CAD build for the part. Positions are in the model's coordinates, mm. A direction names the side the tool comes from. Round coordinates to 2 decimals unless told otherwise and drop trailing zeros. Loops run counter-clockwise (first coordinate to the right, second up) from the corner with the lowest first, then second, coordinate; pieces in that order, holes last. Notation, with made-up numbers: M 17.5,31 L 35.5,31 A15 cw 35.5,46 Z; hole C 88.5,-32 d5. An arc over 180 degrees is marked long. Put each result on its own line as item: value. Start each with the question number.
from build123d import *

# Parameters (mm, degrees)
BOSS_EXTRUDE1_DEPTH      = 15.5
BOSS_EXTRUDE1_DEPTH_BACK = 15.5
SKETCH1_W                = 63.5
SKETCH1_H                = 58.5
SHELL1_T                 = 3
SKETCH2_W                = 16
SKETCH2_H                = 52
CUT_EXTRUDE1_DEPTH       = 39.5
SKETCH3_W                = 53.5
SKETCH3_H                = 31
CUT_EXTRUDE2_DEPTH       = 39.5
BOSS_EXTRUDE2_START      = -15.5
SKETCH4_R                = 1.6
BOSS_EXTRUDE2_DEPTH      = 3
FILLET1_R                = 3.5
FILLET2_R                = 1


with BuildPart() as part:
    # Sketch1 → Boss-Extrude1 (new, two sides: drawn at the far end of the back side and taken through both)
    with BuildSketch(Plane(origin=(0, 0, 0), x_dir=(1, 0, 0), z_dir=(0, 1, 0)).offset(-BOSS_EXTRUDE1_DEPTH_BACK)):
        Rectangle(SKETCH1_W, SKETCH1_H)
    extrude(amount=BOSS_EXTRUDE1_DEPTH + BOSS_EXTRUDE1_DEPTH_BACK)

    # Shell1
    shell1_openings = [part.faces().sort_by_distance(p)[0] for p in [
        (0, -15.5, 0),
    ]]
    offset(amount=SHELL1_T, openings=shell1_openings, kind=Kind.INTERSECTION)

    # Sketch2 → Cut-Extrude1 (cut)
    with BuildSketch(Plane(origin=(0, 18.5, 0), x_dir=(1, 0, 0), z_dir=(0, 1, 0))):
        with Locations((-8.25, 6.25)):
            Rectangle(SKETCH2_W, SKETCH2_H)
    extrude(amount=-CUT_EXTRUDE1_DEPTH, mode=Mode.SUBTRACT)

    # Sketch3 → Cut-Extrude2 (cut)
    with BuildSketch(Plane(origin=(0, 0, -32.25), x_dir=(-1, 0, 0), z_dir=(0, 0, -1))):
        Rectangle(SKETCH3_W, SKETCH3_H)
    extrude(amount=-CUT_EXTRUDE2_DEPTH, mode=Mode.SUBTRACT)

    # Sketch4 → Boss-Extrude2 (add)
    with BuildSketch(Plane(origin=(0, 0, 0), x_dir=(1, 0, 0), z_dir=(0, 1, 0)).offset(BOSS_EXTRUDE2_START)):
        Polygon((-26.75, 32.25), (-26.75, 44), (-39.5, 44), (-39.5, -44), (39.5, -44), (39.5, 44), (26.75, 44), (26.75, 32.25), (34.75, 32.25), (34.75, -32.25), (-34.75, -32.25), (-34.75, 32.25), align=None)
        with Locations(Location((-35.5, 40, 0), (0, 0, 90))):
            Circle(SKETCH4_R, mode=Mode.SUBTRACT)
        with Locations(Location((-35.5, -40, 0), (0, 0, 90))):
            Circle(SKETCH4_R, mode=Mode.SUBTRACT)
        with Locations(Location((35.5, -40, 0), (0, 0, 90))):
            Circle(SKETCH4_R, mode=Mode.SUBTRACT)
        with Locations(Location((35.5, 40, 0), (0, 0, 90))):
            Circle(SKETCH4_R, mode=Mode.SUBTRACT)
    extrude(amount=BOSS_EXTRUDE2_DEPTH)

    # Fillet1
    # the kernel refuses this fillet: 3.5 mm, written as the material it adds along each edge
    with BuildSketch(Plane(origin=(34.75, -12.5, -32.25), x_dir=(1, 0, 0), z_dir=(0, 0, 1)), Plane(origin=(-34.75, -12.5, 32.25), x_dir=(-1, 0, 0), z_dir=(0, 0, -1))) as fillet1_piece_1:
        with BuildLine():
            CenterArc((FILLET1_R, FILLET1_R), FILLET1_R, 180, 90)
            Line((0, FILLET1_R), (0, 0))
            Line((0, 0), (FILLET1_R, 0))
        make_face()
    extrude(amount=64.5)
    with BuildSketch(Plane(origin=(34.75, -12.5, 32.25), x_dir=(0, 0, 1), z_dir=(-1, 0, 0))) as fillet1_piece_2:
        with BuildLine():
            CenterArc((FILLET1_R, FILLET1_R), FILLET1_R, 180, 90)
            Line((0, FILLET1_R), (0, 0))
            Line((0, 0), (FILLET1_R, 0))
        make_face()
    extrude(amount=69.5)
    with BuildSketch(Plane(origin=(34.75, -12.5, -32.25), x_dir=(1, 0, 0), z_dir=(0, 0, 1))) as fillet1_piece_3a_section:
        with BuildLine():
            CenterArc((FILLET1_R, FILLET1_R), FILLET1_R, 180, 90)
            Line((0, FILLET1_R), (0, 0))
            Line((0, 0), (FILLET1_R, 0))
        make_face()
    fillet1_piece_3a = extrude(amount=73.25, mode=Mode.PRIVATE)
    fillet1_piece_3a = fillet1_piece_3a - Plane(origin=(35.5, -12.5, 40), x_dir=(0, 0, -1), z_dir=(0, -1, 0)) * Cylinder(1.6, 161, mode=Mode.PRIVATE)
    fillet1_piece_3a = split(fillet1_piece_3a, bisect_by=Plane(origin=(34.75, -12.5, 32.25), z_dir=(0, 0, 1)), keep=Keep.TOP, mode=Mode.PRIVATE)
    with BuildSketch(Plane(origin=(43.5, -12.5, 32.25), x_dir=(0, 0, 1), z_dir=(-1, 0, 0))) as fillet1_piece_3b_section:
        with BuildLine():
            CenterArc((FILLET1_R, FILLET1_R), FILLET1_R, 180, 90)
            Line((0, FILLET1_R), (0, 0))
            Line((0, 0), (FILLET1_R, 0))
        make_face()
    fillet1_piece_3b = extrude(amount=78.25, mode=Mode.PRIVATE)
    fillet1_piece_3b = split(fillet1_piece_3b, bisect_by=Plane(origin=(39.5, -12.5, 32.25), z_dir=(-1, 0, 0)), keep=Keep.TOP, mode=Mode.PRIVATE)
    fillet1_piece_3b = split(fillet1_piece_3b, bisect_by=Plane(origin=(34.75, -12.5, 32.25), z_dir=(1, 0, 0)), keep=Keep.TOP, mode=Mode.PRIVATE)
    fillet1_piece_3 = fillet1_piece_3a & fillet1_piece_3b
    add(fillet1_piece_3)
    with BuildSketch(Plane(origin=(34.75, -12.5, 32.25), x_dir=(0, 0, 1), z_dir=(-1, 0, 0))) as fillet1_piece_4a_section:
        with BuildLine():
            CenterArc((FILLET1_R, FILLET1_R), FILLET1_R, 180, 90)
            Line((0, FILLET1_R), (0, 0))
            Line((0, 0), (FILLET1_R, 0))
        make_face()
    fillet1_piece_4a = extrude(amount=78.25, mode=Mode.PRIVATE)
    fillet1_piece_4a = split(fillet1_piece_4a, bisect_by=Plane(origin=(-39.5, -12.5, 32.25), z_dir=(1, 0, 0)), keep=Keep.TOP, mode=Mode.PRIVATE)
    fillet1_piece_4a = split(fillet1_piece_4a, bisect_by=Plane(origin=(-34.75, -12.5, 32.25), z_dir=(-1, 0, 0)), keep=Keep.TOP, mode=Mode.PRIVATE)
    with BuildSketch(Plane(origin=(-34.75, -12.5, 41), x_dir=(-1, 0, 0), z_dir=(0, 0, -1))) as fillet1_piece_4b_section:
        with BuildLine():
            CenterArc((FILLET1_R, FILLET1_R), FILLET1_R, 180, 90)
            Line((0, FILLET1_R), (0, 0))
            Line((0, 0), (FILLET1_R, 0))
        make_face()
    fillet1_piece_4b = extrude(amount=73.25, mode=Mode.PRIVATE)
    fillet1_piece_4b = fillet1_piece_4b - Plane(origin=(-35.5, -12.5, 40), x_dir=(0, 0, -1), z_dir=(0, -1, 0)) * Cylinder(1.6, 161, mode=Mode.PRIVATE)
    fillet1_piece_4b = split(fillet1_piece_4b, bisect_by=Plane(origin=(-34.75, -12.5, 32.25), z_dir=(0, 0, 1)), keep=Keep.TOP, mode=Mode.PRIVATE)
    fillet1_piece_4 = fillet1_piece_4a & fillet1_piece_4b
    add(fillet1_piece_4)
    # the kernel refuses this fillet: 3.5 mm, written as the material it takes off along each edge
    with BuildSketch(Plane(origin=(-0.25, 18.5, 19.75), x_dir=(0, 0, 1), z_dir=(-1, 0, 0))) as fillet1_2_piece_1:
        with BuildLine():
            CenterArc((3.464101615, -3.5), FILLET1_R, 90, 81.786789298)
            Line((0, -3), (0, 0))
            Line((0, 0), (3.464101615, 0))
        make_face()
    extrude(amount=16, mode=Mode.SUBTRACT)
    with BuildSketch(Plane(origin=(-0.25, 18.5, -40.910254038), x_dir=(1, 0, 0), z_dir=(0, 0, 1)), Plane(origin=(-16.25, 18.5, 19.75), x_dir=(-1, 0, 0), z_dir=(0, 0, -1))) as fillet1_2_piece_2:
        with BuildLine():
            CenterArc((3.464101615, -3.5), FILLET1_R, 90, 81.786789298)
            Line((0, -3), (0, 0))
            Line((0, 0), (3.464101615, 0))
        make_face()
    extrude(amount=60.660254038, mode=Mode.SUBTRACT)
    with BuildSketch(Plane(origin=(-7.5, 18.5, -32.25), x_dir=(0, 0, 1), z_dir=(-1, 0, 0))) as fillet1_2_piece_3:
        with BuildLine():
            CenterArc((FILLET1_R, -FILLET1_R), FILLET1_R, 90, 90)
            Line((0, -FILLET1_R), (0, 0))
            Line((0, 0), (FILLET1_R, 0))
        make_face()
    extrude(amount=36, mode=Mode.SUBTRACT)
    with BuildSketch(Plane(origin=(43.5, 18.5, -32.25), x_dir=(0, 0, 1), z_dir=(-1, 0, 0))) as fillet1_2_piece_4:
        with BuildLine():
            CenterArc((FILLET1_R, -FILLET1_R), FILLET1_R, 90, 90)
            Line((0, -FILLET1_R), (0, 0))
            Line((0, 0), (FILLET1_R, 0))
        make_face()
    extrude(amount=52.5, mode=Mode.SUBTRACT)
    with BuildSketch(Plane(origin=(-34.75, 18.5, 41), x_dir=(0, -1, 0), z_dir=(0, 0, -1))) as fillet1_2_piece_5:
        with BuildLine():
            CenterArc((FILLET1_R, -FILLET1_R), FILLET1_R, 90, 90)
            Line((0, -FILLET1_R), (0, 0))
            Line((0, 0), (FILLET1_R, 0))
        make_face()
    extrude(amount=82, mode=Mode.SUBTRACT)
    with BuildSketch(Plane(origin=(34.75, 18.5, 41), x_dir=(0, -1, 0), z_dir=(0, 0, -1))) as fillet1_2_piece_6:
        with BuildLine():
            CenterArc((FILLET1_R, FILLET1_R), FILLET1_R, 180, 90)
            Line((0, FILLET1_R), (0, 0))
            Line((0, 0), (FILLET1_R, 0))
        make_face()
    extrude(amount=82, mode=Mode.SUBTRACT)
    with BuildSketch(Plane(origin=(-43.5, 18.5, 32.25), x_dir=(0, -1, 0), z_dir=(1, 0, 0))) as fillet1_2_piece_7:
        with BuildLine():
            CenterArc((FILLET1_R, FILLET1_R), FILLET1_R, 180, 90)
            Line((0, FILLET1_R), (0, 0))
            Line((0, 0), (FILLET1_R, 0))
        make_face()
    extrude(amount=87, mode=Mode.SUBTRACT)
    with BuildSketch(Plane(origin=(8.410254038, 18.5, 19.75), x_dir=(0, 0, 1), z_dir=(-1, 0, 0))) as fillet1_2_piece_8a_section:
        with BuildLine():
            CenterArc((3.464101615, -3.5), FILLET1_R, 90, 81.786789298)
            Line((0, -3), (0, 0))
            Line((0, 0), (3.464101615, 0))
        make_face()
    fillet1_2_piece_8a = extrude(amount=24.660254038, mode=Mode.PRIVATE)
    fillet1_2_piece_8a = split(fillet1_2_piece_8a, bisect_by=Plane(origin=(-0.25, 18.5, 19.75), z_dir=(1, 0, 0)), keep=Keep.TOP, mode=Mode.PRIVATE)
    with BuildSketch(Plane(origin=(-0.25, 18.5, -32.25), x_dir=(1, 0, 0), z_dir=(0, 0, 1))) as fillet1_2_piece_8b_section:
        with BuildLine():
            CenterArc((3.464101615, -3.5), FILLET1_R, 90, 81.786789298)
            Line((0, -3), (0, 0))
            Line((0, 0), (3.464101615, 0))
        make_face()
    fillet1_2_piece_8b = extrude(amount=60.660254038, mode=Mode.PRIVATE)
    fillet1_2_piece_8b = split(fillet1_2_piece_8b, bisect_by=Plane(origin=(-0.25, 18.5, 19.75), z_dir=(0, 0, 1)), keep=Keep.TOP, mode=Mode.PRIVATE)
    fillet1_2_piece_8 = fillet1_2_piece_8a & fillet1_2_piece_8b
    add(fillet1_2_piece_8, mode=Mode.SUBTRACT)
    with BuildSketch(Plane(origin=(-16.25, 18.5, 28.410254038), x_dir=(-1, 0, 0), z_dir=(0, 0, -1))) as fillet1_2_piece_9a_section:
        with BuildLine():
            CenterArc((3.464101615, -3.5), FILLET1_R, 90, 81.786789298)
            Line((0, -3), (0, 0))
            Line((0, 0), (3.464101615, 0))
        make_face()
    fillet1_2_piece_9a = extrude(amount=60.660254038, mode=Mode.PRIVATE)
    fillet1_2_piece_9a = split(fillet1_2_piece_9a, bisect_by=Plane(origin=(-16.25, 18.5, 19.75), z_dir=(0, 0, 1)), keep=Keep.TOP, mode=Mode.PRIVATE)
    with BuildSketch(Plane(origin=(-0.25, 18.5, 19.75), x_dir=(0, 0, 1), z_dir=(-1, 0, 0))) as fillet1_2_piece_9b_section:
        with BuildLine():
            CenterArc((3.464101615, -3.5), FILLET1_R, 90, 81.786789298)
            Line((0, -3), (0, 0))
            Line((0, 0), (3.464101615, 0))
        make_face()
    fillet1_2_piece_9b = extrude(amount=24.660254038, mode=Mode.PRIVATE)
    fillet1_2_piece_9b = split(fillet1_2_piece_9b, bisect_by=Plane(origin=(-16.25, 18.5, 19.75), z_dir=(-1, 0, 0)), keep=Keep.TOP, mode=Mode.PRIVATE)
    fillet1_2_piece_9 = fillet1_2_piece_9a & fillet1_2_piece_9b
    add(fillet1_2_piece_9, mode=Mode.SUBTRACT)

    # Fillet2
    fillet2_edges = [part.edges().sort_by_distance(p)[0] for p in [
        (26.75, -12.5, -38.125),
        (32.5, -12.5, -32.25),
        (-32.5, -12.5, -32.25),
        (-26.75, -12.5, -38.125),
        (-33.125, -12.5, -44),
        (-39.5, -12.5, 0),
        (0, -12.5, 44),
        (39.5, -12.5, 0),
        (33.125, -12.5, -44),
        (-26.75, 15.250643519, -32.241013868),
        (26.75, 1.25, -32.25),
        (26.75, 15.250643519, -32.241013868),
        (-26.75, 1.25, -32.25),
    ]]
    fillet(fillet2_edges, radius=FILLET2_R)


solid = part.part
(1) Cut at C-C on x = 23.5. List the corners of the cut face in (y, z), and give its area (3 significant figures).
(2) Cut at A-A on z = -40. List the corners of the cut face in (x, y).
(3) Mould opens along X. For faces 1 (the flat face through (-29, 0, -29.25)), 2 (the cylindrical face through (-35.7, -11.4, 1.7)), 3 (the flat face through (7, 18.5, 0)), 4 (the cylindrical face through (36.92, -14.02, -40.74)) say: +X half, -X half, draft (parallel to the pull), parting line (faces both ways), or undercut.
(4) Cut at D-D on z = 40. List the corners of the cut face in (x, y).
(5) Flat gauge pins, fed straight in: pin 1 Ø4 at (x, z) = (-35.5, 40) entering from +Y; pin 2 Ø4 at (x, y) = (30.5, 1) entering from +Z; pin 3 Ø6 at (x, z) = (21, -25) entering from -Y; pin 4 Ø12 at (x, y) = (-30.5, -10) entering from -Z. Where does each tip first touch, or does it go through?
(6) Tool access for faces 5 (the cylindrical face through (-8.09, 17.67, 20.95)), 6 (the flat face through (-31.75, 0, 0)), 7 (the flat face through (-26.75, -4, -31)), 8 (the cylindrical face through (-0.5, 17.5, 31.2)): list every direction of +Z, -Z, +X, -X, +Y, -Y with a clear straight run to the whole face (end or side of a thin tool).
(7) Cut at B-B on z = 11. List the corners of the cut face in (x, y), and give its area (3 significant figures).
(8) Drill centre lines: line 1 along Z through (x, y) = (35.5, -14.25); line 2 along X through (y, z) = (2.5, 29); line 3 along X through (y, z) = (13, -30.5). Where is each one in solid material? Low to high.
Taken from the geometry:
1. outline: M -15.5,29.25 L 15.5,29.25 L 15.5,-32.21 A3.5 ccw 18.5,-28.75 L 18.5,28.75 A3.5 ccw 15,32.25 L -9,32.25 A3.5 cw -12.5,35.75 L -12.5,43 A1 ccw -13.5,44 L -15.5,44 Z
1. area: 319 mm2
2. outline: M -39.5,-15.5 L -37.1,-15.5 L -37.1,-12.5 L -38.5,-12.5 A1 ccw -39.5,-13.5 Z; M -33.9,-15.5 L -26.75,-15.5 L -26.75,-13.5 A1 ccw -27.75,-12.5 L -33.9,-12.5 Z; M 26.75,-15.5 L 33.9,-15.5 L 33.9,-12.5 L 27.75,-12.5 A1 ccw 26.75,-13.5 Z; M 37.1,-15.5 L 39.5,-15.5 L 39.5,-13.5 A1 ccw 38.5,-12.5 L 37.1,-12.5 Z
3. face 1: undercut
3. face 2: -X half
3. face 3: draft
3. face 4: undercut
4. outline: M -39.5,-15.5 L -37.1,-15.5 L -37.1,-12.5 L -38.5,-12.5 A1 ccw -39.5,-13.5 Z; M -33.9,-15.5 L 33.9,-15.5 L 33.9,-12.5 L -33.9,-12.5 Z; M 37.1,-15.5 L 39.5,-15.5 L 39.5,-13.5 A1 ccw 38.5,-12.5 L 37.1,-12.5 Z
5. pin 1: y = -12.5
5. pin 2: z = 32.25
5. pin 3: y = 15.5
5. pin 4: z = -44
6. face 5: -Z, +Y
6. face 6: -Y
6. face 7: -Z, -Y
6. face 8: +Z, +X, -X, +Y
7. outline: M -39.5,-15.5 L -31.75,-15.5 L -31.75,15.5 L -16.25,15.5 A3.5 ccw -19.71,18.5 L -31.25,18.5 A3.5 ccw -34.75,15 L -34.75,-9 A3.5 cw -38.25,-12.5 L -38.5,-12.5 A1 ccw -39.5,-13.5 Z; M -0.25,15.5 L 31.75,15.5 L 31.75,-15.5 L 39.5,-15.5 L 39.5,-13.5 A1 ccw 38.5,-12.5 L 38.25,-12.5 A3.5 cw 34.75,-9 L 34.75,15 A3.5 ccw 31.25,18.5 L 3.21,18.5 A3.5 ccw Z
7. area: 370 mm2
8. line 1: -44 to -41.6, -38.4 to 38.4, 41.6 to 44
8. line 2: -34.75 to -31.75, 31.75 to 34.75
8. line 3: -34.75 to -26.75, 26.75 to 34.75
